```python
from build123d import *

# Parameters (mm, degrees)
CROQUIS1_R              = 45
CROQUIS1_R_2            = 40.5
CROQUIS1_R_3            = 17.3
CROQUIS1_R_4            = 13.5
SALIENTE_EXTRUIR1_DEPTH = 2
CROQUIS2_R              = 45
SALIENTE_EXTRUIR2_DEPTH = 2
CROQUIS3_R              = 56.484635106
CROQUIS3_R_2            = 40.5
CORTAR_EXTRUIR1_DEPTH   = 10
REDONDEO2_R             = 1.5


with BuildPart() as part:
    # Croquis1 → Saliente-Extruir1 (new body)
    with BuildSketch(Plane(origin=(0, 0, 0), x_dir=(1, 0, 0), z_dir=(0, 1, 0))):
        Circle(CROQUIS1_R)
        Circle(CROQUIS1_R_2, mode=Mode.SUBTRACT)
        Circle(CROQUIS1_R_2)
        Circle(CROQUIS1_R_3, mode=Mode.SUBTRACT)
        Circle(CROQUIS1_R_4)
    extrude(amount=SALIENTE_EXTRUIR1_DEPTH)

    # Croquis2 → Saliente-Extruir2 (add)
    with BuildSketch(Plane.XZ):
        Circle(CROQUIS2_R)
    extrude(amount=SALIENTE_EXTRUIR2_DEPTH)

    # Croquis3 → Cortar-Extruir1 (cut)
    with BuildSketch(Plane(origin=(0, 2, 0), x_dir=(1, 0, 0), z_dir=(0, 1, 0))):
        Circle(CROQUIS3_R)
        Circle(CROQUIS3_R_2, mode=Mode.SUBTRACT)
    extrude(amount=-CORTAR_EXTRUIR1_DEPTH, mode=Mode.SUBTRACT)

    # Redondeo2
    redondeo2_edges = [part.edges().sort_by_distance(p)[0] for p in [
        (-13.5, 2, 0),
        (-40.5, 2, 0),
        (-17.3, 2, 0),
    ]]
    fillet(redondeo2_edges, radius=REDONDEO2_R)


solid = part.part
```
The model under review builds one solid part; all positions refer to its coordinate system, in mm. A direction names the side the tool comes from. Round coordinates to 2 decimals unless told otherwise and drop trailing zeros. Loops run counter-clockwise (first coordinate to the right, second up) from the corner with the lowest first, then second, coordinate; pieces in that order, holes last.
Item 1: Take a section at A-A (x = 0). Write out the cut boundary in (y, z).
Determined:
outline: (-2, -40.5) - (0.5, -40.5) arc R1.5 ccw to (2, -39) - (2, -18.8) arc R1.5 ccw to (0.5, -17.3) - (0, -17.3) - (0, -13.5) - (0.5, -13.5) arc R1.5 ccw to (2, -12) - (2, 12) arc R1.5 ccw to (0.5, 13.5) - (0, 13.5) - (0, 17.3) - (0.5, 17.3) arc R1.5 ccw to (2, 18.8) - (2, 39) arc R1.5 ccw to (0.5, 40.5) - (-2, 40.5) - close
Item 2: For line 1 (Z direction, x = 0, y = 0.35); line 2 (X direction, y = 1.1, z = 8.5), list the stretches that pass through material, from the lowest coordinate up.
Determined:
line 1: z = -40.5 to -17.3, -13.5 to 13.5, 17.3 to 40.5
line 2: x = -39.47 to -15.21, -10.33 to 10.33, 15.21 to 39.47
Item 3: Take a section at B-B (z = 0). Write out the cut boundary in (x, y), then the cut area to 3 significant figures.
Determined:
outline: (-40.5, -2) - (40.5, -2) - (40.5, 0.5) arc R1.5 ccw to (39, 2) - (18.8, 2) arc R1.5 ccw to (17.3, 0.5) - (17.3, 0) - (13.5, 0) - (13.5, 0.5) arc R1.5 ccw to (12, 2) - (-12, 2) arc R1.5 ccw to (-13.5, 0.5) - (-13.5, 0) - (-17.3, 0) - (-17.3, 0.5) arc R1.5 ccw to (-18.8, 2) - (-39, 2) arc R1.5 ccw to (-40.5, 0.5) - close
area: 306 mm2
Item 4: Mouldability with a two-part tool opening along Z and no side actions: class faces 1 (the face through (-9.1, 0, -10.2)), 2 (the face through (21.77, -0.73, -34.15)), 3 (the face through (0, 2, 0)) as released by +Z, released by -Z, zero draft, split by the parting line, or undercut.
Determined:
face 1: undercut
face 2: split by the parting line
face 3: zero draft
Item 5: For faces 4 (the face through (16.5, 0.2, -5.2)), 5 (the face through (-1, -2, 1)), list the 3-axis set-ups (+Z, -Z, +X, -X, +Y, -Y) from which the entire face can be reached by the end or side of a thin tool; tool diameter is ignored.
Determined:
face 4: +Y
face 5: +Z, -Z, +X, -X, -Y
Item 6: Clearance check with a flat-ended pin moving along its axis: pin 1 Ø2 at (y, z) = (0, 20.5) entering from -X. State where the tip first meets the part, or that it passes through.
Determined:
pin 1: stops at x = -35.5
